Verification items for the finished model (mm, model axes). A direction names the side the tool comes from. Coordinates: 2 decimals unless noted, no trailing zeros. Loops run counter-clockwise (first coordinate to the right, second up) from the corner with the lowest first, then second, coordinate; pieces in that order, holes last. Notation, with made-up numbers: (-31, 60) - (16, 60) arc R25 cw to (16, 99) - close; hole circle Ø9 at (0.25, 80.25). An arc over 180 degrees is marked (long way). One line per item, written item: value. Start each with the question number.
(1) Set-up check for faces 1 (the face through (60, 1, -250)), 2 (the face through (60.538, 70, -123)), 3 (the face through (60.538, -70, -123)): record each of +Z, -Z, +X, -X, +Y, -Y from which the full face is reachable in a straight line by a thin tool's end or side.
(2) Gauge pin test, flat ends, axial feed: P1, Ø1, axis at x = 62, z = -153, coming from the +Y side; P2, Ø0.6, axis at x = 61.5, z = -105, coming from the -Y side; P3, Ø1.4, axis at y = -71, z = -133.5, coming from the +X side. Record the tip position at first contact, or that the pin passes through.
(3) Section check B-B (x = 61.35). Record the boundary of the cut face in (y, z).
(4) Thickness scan on probe 1 along Y at (x, z) = (61.05, -196.5). Record the ranges inside material, lowest first. Write a range as [from, to].
(5) Section check A-A (z = -141.5). Record the boundary of the cut face in (x, y).
Autodesk Inventor part; units mm, degrees
ref_plane "Work Plane2" through (-62.538, -75, -250) normal (0, 0, 1) x (1, 0, 0)
ref_plane "YZ Plane" through (0, 0, 0) normal (1, 0, 0) x (0, 1, 0)
ref_plane "XZ Plane" through (0, 0, 0) normal (0, 1, 0) x (-1, 0, 0)
ref_plane "Work Plane1" through (0, 0, 0) normal (0, 0, 1) x (1, 0, 0)
sketch "Sketch1" plane through (0, 0, 0) normal (0, 0, 1) x (1, 0, 0)
  line L0 (62.538, -67.5) -> (62.538, 67.5)
  line L1 (57.538, 75) -> (57.538, -75)
  line L2 (60.538, 72.3) -> (57.538, 72.3)
  line L3 (60.538, 67.5) -> (60.538, 72.5)
  line L4 (60.538, -72.3) -> (57.538, -72.3)
  line L5 (60.538, -72.5) -> (60.538, -67.5)
  line L6 (62.538, -67.5) -> (60.538, -67.5)
  line L7 (57.538, 72.3) -> (60.538, 72.3)
  line L8 (60.538, 72.3) -> (60.538, -72.3)
  line L9 (60.538, -72.3) -> (57.538, -72.3)
  line L10 (57.538, -72.3) -> (57.538, 72.3)
  line L11 (62.538, -67.5) -> (60.538, -67.5)
  line L12 (60.538, -67.5) -> (60.538, 67.5)
  line L13 (60.538, 67.5) -> (62.538, 67.5)
  line L14 (62.538, 67.5) -> (62.538, -67.5)
  spline S0 degree 3 poles (88.1745, 80.1336) (86.4644, 80.1539) (84.1903, 80.1768) (79.3721, 80.2194) (76.1158, 80.2429) (70.2528, 80.2817) (68.432, 80.2919) (65.9587, 80.3052) knots 0.050371 0.050371 0.050371 0.050371 3.844611 3.844611 8.630626 8.630626 13.703565 13.703565 13.703565 13.703565
  point P0 (0, 0)
  point P1 (62.538, 67.5)
  point P2 (57.538, 72.3)
  point P3 (57.538, -72.3)
ref_plane "Work Plane2" through (-62.538, -75, -250) normal (0, 0, 1) x (1, 0, 0)
extrude "Extrusion1" add sketch "Sketch1" against normal up to surface (250 mm away)
equation "\"BendRadius\" = Thickness"
equation "\"BendReliefWidth\" = Thickness"
equation "\"BendReliefDepth\" = 0.5 * Thickness"
equation "\"CornerReliefSize\" = 4 * Thickness"
equation "\"MinimumRemnant\" = 2 * Thickness"
equation "\"TransitionRadius\" = BendRadius"
equation "\"JacobiRadiusSize\" = BendRadius"
equation "\"GapSize\" = Thickness"
properties part number "Lid1" material "Plastic, Opaque White"
Responses:
1. face 1: -Z, +X, -X, +Y, -Y
1. face 2: +Z, -Z, +X, +Y
1. face 3: +Z, -Z, +X, -Y
2. P1: stops at y = 67.5
2. P2: stops at y = -67.5
2. P3: stops at x = 60.54
3. outline: (-67.5, -250) - (67.5, -250) - (67.5, 0) - (-67.5, 0) - close
4. probe 1: y = [-67.5, 67.5]
5. outline: (57.54, -72.3) - (60.54, -72.3) - (60.54, -67.5) - (62.54, -67.5) - (62.54, 67.5) - (60.54, 67.5) - (60.54, 72.3) - (57.54, 72.3) - close
